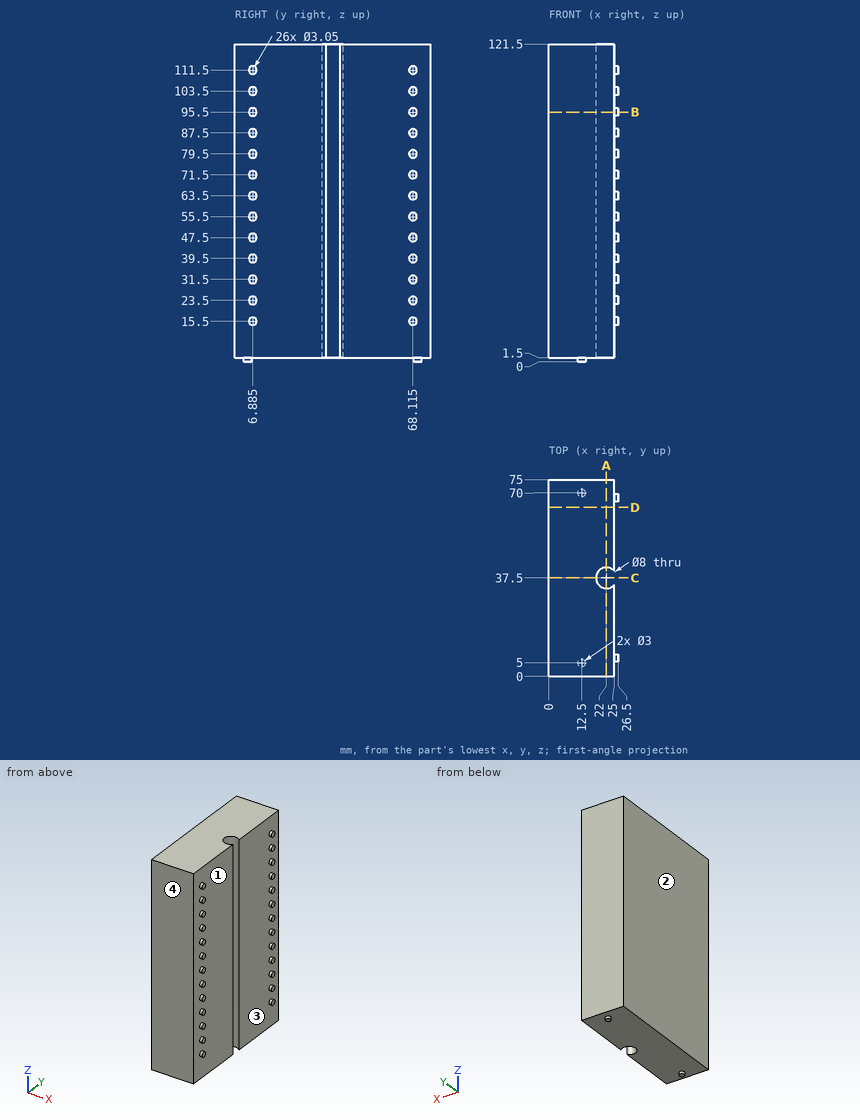
The figure shows three views and two pictorial views of one solid part (mm, origin at its lowest corner). Answer the questions. Coordinates: 2 decimals unless noted, no trailing zeros. Order: outer loops, then holes, each group sorted by start corner. A loop starts at its lowest first (then second) coordinate and runs counter-clockwise, first axis right, second up.
Q1. A cutting plane is placed at D-D, the plane y = 64.5. Write down the section's boundary in (x, z).
Q2. A cutting plane is placed at A-A, the plane x = 22. Write down the section's boundary in (y, z), and give its area (3 significant figures).
Q3. A cutting plane is placed at C-C, the plane y = 37.5. Write down the section's boundary in (x, z).
Q4. For a pull along Y with two mould halves and no side action, classify the marked faces 1, 2, 3 and 4 as pulls with the +Y half, pulls with the -Y half, needs draft (parallel to the pull), parting line crosses it, or undercut.
Q5. A cutting plane is placed at B-B, the plane z = 95.5. Write down the section's boundary in (x, y), and give its area (3 significant figures).
Q6. Consider line 1 (Y direction, x = 22, z = 88); line 2 (X direction, y = 49, z = 112); line 3 (Z direction, x = 22.25, y = 31.5). Determine where each line is inside the solid, lowest interval first.
Q7. Given P1, Ø1.5, axis at x = 14.5, z = 46.5, coming from the -Y side; P2, Ø7.5, axis at x = 9.5, y = 40, coming from the -Z side; P3, Ø17.5, axis at y = 52, z = 70, coming from the +X side, each flat-ended and moving along its own axis, determine where each tip first touches the part or whether it passes through.
Answers follow:
1. outline: (0, 1.5) - (25, 1.5) - (25, 121.5) - (0, 121.5) - close
2. outline: (0, 1.5) - (33.5, 1.5) - (33.5, 121.5) - (0, 121.5) - close; (41.5, 1.5) - (75, 1.5) - (75, 121.5) - (41.5, 121.5) - close
2. area: 8,040 mm2
3. outline: (0, 1.5) - (18, 1.5) - (18, 121.5) - (0, 121.5) - close
4. face 1: undercut
4. face 2: needs draft
4. face 3: undercut
4. face 4: pulls with the -Y half
5. outline: (0, 0) - (25, 0) - (25, 5.36) - (26.5, 5.36) - (26.5, 8.41) - (25, 8.41) - (25, 34.85) arc R4 cw (long way) to (25, 40.15) - (25, 66.59) - (26.5, 66.59) - (26.5, 69.64) - (25, 69.64) - (25, 75) - (0, 75) - close
5. area: 1,840 mm2
6. line 1: y = 0 to 33.5, 41.5 to 75
6. line 2: x = 0 to 25
6. line 3: z = 1.5 to 121.5
7. P1: stops at y = 0
7. P2: stops at z = 1.5
7. P3: stops at x = 25
